Input: part model. Units: mm. Frame: model coordinates. A direction names the side the tool comes from. Round coordinates to 2 decimals unless told otherwise and drop trailing zeros. Loops run counter-clockwise (first coordinate to the right, second up) from the corner with the lowest first, then second, coordinate; pieces in that order, holes last. Notation, with made-up numbers: (73.25, 0.25) - (100.25, 0.25) arc R11 cw to (100.25, 16.25) - close; hole circle Ø1 at (27.25, -3). An arc over 180 degrees is marked (long way). Write each question's results on one line, items separated by ' | '.
from build123d import *

# Parameters (mm, degrees)
F0_R     = 26
F1_DEPTH = 11
F2_T     = -1.8
F3_SIZE  = 0.5


with BuildPart() as f1:
    # F0 (on Top) → F1 (new body)
    with BuildSketch(Plane.XY):
        Circle(F0_R)
    extrude(amount=F1_DEPTH)

    # F2
    f2_openings = [f1.faces().sort_by_distance(p)[0] for p in [
        (0, 0, 11),
    ]]
    offset(amount=F2_T, openings=f2_openings)

    # F3
    f3_edges = [f1.edges().sort_by_distance(p)[0] for p in [
        (-24.2, 0, 11),
    ]]
    chamfer(f3_edges, length=F3_SIZE)


solid = f1.part
1. Section query C-C, the plane z = 1. Output: boundary loops of the cut face in (x, y).
Answer:
outline: circle Ø52 at (0, 0)
2. Line query: line 1 (Y direction, x = 0, z = 5.5); line 2 (Z direction, x = 23, y = -4); line 3 (Y direction, x = 21, z = 6.75). Output: solid intervals per line, ascending. Write a range as [from, to].
Answer:
line 1: [-26, -24.2], [24.2, 26] | line 2: [0, 1.8] | line 3: [-15.33, -12.03], [12.03, 15.33]
3. Mould query, pull axis X, two halves, no side actions, for faces 1 (the flat face through (0, 0, 0)), 2 (the flat face through (0, 0, 1.8)), 3 (the cylindrical face through (-20.633, -15.821, 5.423)). Classes: pulls with the +X half, pulls with the -X half, needs draft (parallel to the pull), parting line crosses it, or undercut.
Answer:
face 1: needs draft | face 2: undercut | face 3: parting line crosses it
4. Contact query for flat-ended pins moving along their axis: pin 1 (4 mm diameter, centred on y = -13.5, z = 4, fed in from -X); pin 2 (3 mm diameter, centred on x = 14, z = 8.5, fed in from -Y); pin 3 (3 mm diameter, centred on y = 16, z = 7.5, fed in from -X); pin 4 (8 mm diameter, centred on x = 9, y = -2, fed in from -Z). Output: stop coordinate, or through.
Answer:
pin 1: x = -23.32 | pin 2: y = -22.8 | pin 3: x = -21.58 | pin 4: z = 0
5. Section query A-A, the plane y = 0. Output: boundary loops of the cut face in (x, z), plus the area to 3 significant figures.
Answer:
outline: (-26, 0) - (26, 0) - (26, 11) - (24.7, 11) - (24.2, 10.5) - (24.2, 1.8) - (-24.2, 1.8) - (-24.2, 10.5) - (-24.7, 11) - (-26, 11) - close | area: 126 mm^2
6. Set-up query: faces 4 (the flat face through (23, -10, 11)), 5 (the cylindrical face through (22.355, -9.269, 6.089)). Return all of +Z, -Z, +X, -X, +Y, -Y with unobstructed straight access to the full face (end or side cutting, diameter ignored); none if empty.
Answer:
face 4: +Z, +X, -X, +Y, -Y | face 5: +Z
